from build123d import *

# Parameters (mm, degrees)
SKETCH_1_W               = 85
SKETCH_1_H               = 300
EXTRUDE_1_DEPTH          = 820
SKETCH_2_W               = 77.5
SKETCH_2_H               = 273
CUT_EXTRUDE_1_DEPTH      = 878.282736636
SKETCH_5_W               = 50
SKETCH_5_H               = 140
EXTRUDE_3_DEPTH          = 11
SKETCH_6_W               = 80
SKETCH_6_H               = 158
EXTRUDE_4_DEPTH          = 18
SKETCH_8_R               = 13
CUT_EXTRUDE_3_DEPTH      = 884.600022635
MIRROR_4_COPY_1_SKETCH_W = 50
MIRROR_4_COPY_1_SKETCH_H = 140
MIRROR_4_COPY_1_DEPTH    = 11
MIRROR_4_COPY_2_SKETCH_W = 80
MIRROR_4_COPY_2_SKETCH_H = 158
MIRROR_4_COPY_2_DEPTH    = 18
MIRROR_4_COPY_3_SKETCH_R = 13
MIRROR_4_COPY_3_DEPTH    = 884.600022635


with BuildPart() as part:
    # 草图1 → 凸台-拉伸1 (new body)
    with BuildSketch(Plane.XY):
        with Locations((42.5, 150)):
            Rectangle(SKETCH_1_W, SKETCH_1_H)
    extrude(amount=EXTRUDE_1_DEPTH)

    # 草图2 → 切除-拉伸1 (cut, through all)
    with BuildSketch(Plane.XY.offset(820)):
        with Locations((46.25, 150)):
            Rectangle(SKETCH_2_W, SKETCH_2_H)
    extrude(amount=-CUT_EXTRUDE_1_DEPTH, mode=Mode.SUBTRACT)

    # 草图5 → 凸台-拉伸3 (add)
    with BuildSketch(Plane.XZ.offset(-286.5)):
        with Locations((46.25, 70)):
            Rectangle(SKETCH_5_W, SKETCH_5_H)
    extrude_3 = extrude(amount=EXTRUDE_3_DEPTH)

    # 草图6 → 凸台-拉伸4 (add)
    with BuildSketch(Plane(origin=(0, 300, 0), x_dir=(1, 0, 0), z_dir=(0, 1, 0))):
        with Locations((42.5, -61)):
            Rectangle(SKETCH_6_W, SKETCH_6_H)
    extrude_4 = extrude(amount=EXTRUDE_4_DEPTH)

    # 草图8 → 切除-拉伸3 (cut, through all)
    with BuildSketch(Plane(origin=(0, 318, 0), x_dir=(1, 0, 0), z_dir=(0, 1, 0))):
        with Locations(Location((42.5, -20, 0), (0, 0, 270))):
            Circle(SKETCH_8_R)
        with Locations(Location((42.5, -100, 0), (0, 0, 270))):
            Circle(SKETCH_8_R)
    cut_extrude_3 = extrude(amount=-CUT_EXTRUDE_3_DEPTH, mode=Mode.SUBTRACT)

    # 镜向3: 凸台-拉伸3, 凸台-拉伸4, 切除-拉伸3 across plane
    add(extrude_3.mirror(Plane(origin=(0, 150, 0), x_dir=(0, 0, 1), z_dir=(0, -1, 0))))
    add(extrude_4.mirror(Plane(origin=(0, 150, 0), x_dir=(0, 0, 1), z_dir=(0, -1, 0))))
    add(cut_extrude_3.mirror(Plane(origin=(0, 150, 0), x_dir=(0, 0, 1), z_dir=(0, -1, 0))), mode=Mode.SUBTRACT)

    # 镜向4: 凸台-拉伸3, 凸台-拉伸4, 切除-拉伸3 across plane
    add(extrude_3.mirror(Plane(origin=(0, 0, 410), x_dir=(1, 0, 0), z_dir=(0, 0, -1))))
    add(extrude_4.mirror(Plane(origin=(0, 0, 410), x_dir=(1, 0, 0), z_dir=(0, 0, -1))))
    add(cut_extrude_3.mirror(Plane(origin=(0, 0, 410), x_dir=(1, 0, 0), z_dir=(0, 0, -1))), mode=Mode.SUBTRACT)

    # 镜向4 copy 1 sketch → 镜向4 copy 1 (add)
    with BuildSketch(Plane(origin=(0, 13.5, 820), x_dir=(1, 0, 0), z_dir=(0, 1, 0))):
        with Locations((46.25, 70)):
            Rectangle(MIRROR_4_COPY_1_SKETCH_W, MIRROR_4_COPY_1_SKETCH_H)
    extrude(amount=MIRROR_4_COPY_1_DEPTH)

    # 镜向4 copy 2 sketch → 镜向4 copy 2 (add)
    with BuildSketch(Plane(origin=(0, 0, 820), x_dir=(1, 0, 0), z_dir=(0, -1, 0))):
        with Locations((42.5, -61)):
            Rectangle(MIRROR_4_COPY_2_SKETCH_W, MIRROR_4_COPY_2_SKETCH_H)
    extrude(amount=MIRROR_4_COPY_2_DEPTH)

    # 镜向4 copy 3 sketch → 镜向4 copy 3 (cut, through all)
    with BuildSketch(Plane(origin=(0, -18, 820), x_dir=(1, 0, 0), z_dir=(0, -1, 0))):
        with Locations(Location((42.5, -20, 0), (0, 0, 270))):
            Circle(MIRROR_4_COPY_3_SKETCH_R)
        with Locations(Location((42.5, -100, 0), (0, 0, 270))):
            Circle(MIRROR_4_COPY_3_SKETCH_R)
    extrude(amount=-MIRROR_4_COPY_3_DEPTH, mode=Mode.SUBTRACT)


solid = part.part
Geometry: final body of the model. Coordinates: model frame, mm. A direction names the side the tool comes from. Give positions to 0.01 mm unless a question says otherwise; leave off trailing zeros. Loops run counter-clockwise (first coordinate to the right, second up) from the corner with the lowest first, then second, coordinate; pieces in that order, holes last. Notation, with made-up numbers: (63.25, 56) - (115.25, 56) arc R16 ccw to (115.25, 65) - close; hole circle Ø11 at (61.25, 32.5). An arc over 180 degrees is marked (long way). One line per question, with ' | ' between items. Start each with the question number.
(1) Section query D-D on z = 52. Return loops of the section in (x, y).
(2) Reachability of faces 5 (the flat face through (42, 309, 680)), 6 (the flat face through (82.5, 309, 62)), 7 (the flat face through (42, 0, 829)), 8 (the flat face through (46, 275.5, 71)), 9 (the flat face through (2.5, 309, 62)) from +Z, -Z, +X, -X, +Y, -Y: full face, straight path, thin tool, end or side. Return the list, or none.
(3) Section query C-C on y = 143.5. Return loops of the section in (x, z), then the cut area to 3 significant figures.
(4) Section query A-A on z = 800. Count the separate pieces of the cut face and the enclosed holes in it, then the cut area to 3 significant figures.
(5) Contact query for flat-ended pins moving along their axis: pin 1 (9 mm diameter, centred on x = 54, y = 281.5, fed in from +Z); pin 2 (12 mm diameter, centred on y = 232.5, z = 101, fed in from +X); pin 3 (4 mm diameter, centred on y = 25, z = 116, fed in from +X); pin 4 (21 mm diameter, centred on x = 42.5, z = 720, fed in from +Y). Output: stop coordinate, or through.
(6) Ray query, line 1 (Z direction, x = 42, y = 287); line 2 (Y direction, x = 62.5, z = 281); line 3 (X direction, y = 303, z = 100). Return the intervals inside material, ascending. Write a range as from..to.
(7) Section query B-B on z = 436. Return loops of the section in (x, y), then the cut area to 3 significant figures.
(8) Pull-direction query (Z, two-part tool) for faces 1 (the cylindrical face through (46.4, 3, 787.6)), 2 (the flat face through (42, 309, -18)), 3 (the flat face through (42, -9, 140)), 4 (the flat face through (42, 300, 829)); classes: released by +Z, released by -Z, zero draft, split by the parting line, or undercut.
The answers:
1) outline: (0, 0) - (2.5, 0) - (2.5, -18) - (82.5, -18) - (82.5, 0) - (85, 0) - (85, 13.5) - (71.25, 13.5) - (71.25, 24.5) - (21.25, 24.5) - (21.25, 13.5) - (7.5, 13.5) - (7.5, 286.5) - (21.25, 286.5) - (21.25, 275.5) - (71.25, 275.5) - (71.25, 286.5) - (85, 286.5) - (85, 300) - (82.5, 300) - (82.5, 318) - (2.5, 318) - (2.5, 300) - (0, 300) - close
2) face 5: +X, -X, +Y | face 6: +Z, -Z, +X, +Y | face 7: +Z, +X, -X | face 8: +Z, -Z, +X | face 9: +Z, -Z, -X, +Y
3) outline: (0, 0) - (7.5, 0) - (7.5, 820) - (0, 820) - close | area: 6,150 mm2
4) separate pieces: 3 | enclosed holes: 0 | area: 6,110 mm2
5) pin 1: z = 820 | pin 2: x = 7.5 | pin 3: x = 71.25 | pin 4: through
6) line 1: 0..7.01, 32.99..87.01, 112.99..707.01, 732.99..787.01, 812.99..820 | line 2: 0..13.5, 286.5..300 | line 3: 2.5..29.5, 55.5..82.5
7) outline: (0, 0) - (85, 0) - (85, 13.5) - (7.5, 13.5) - (7.5, 286.5) - (85, 286.5) - (85, 300) - (0, 300) - close | area: 4,340 mm2
8) face 1: undercut | face 2: released by -Z | face 3: undercut | face 4: zero draft
